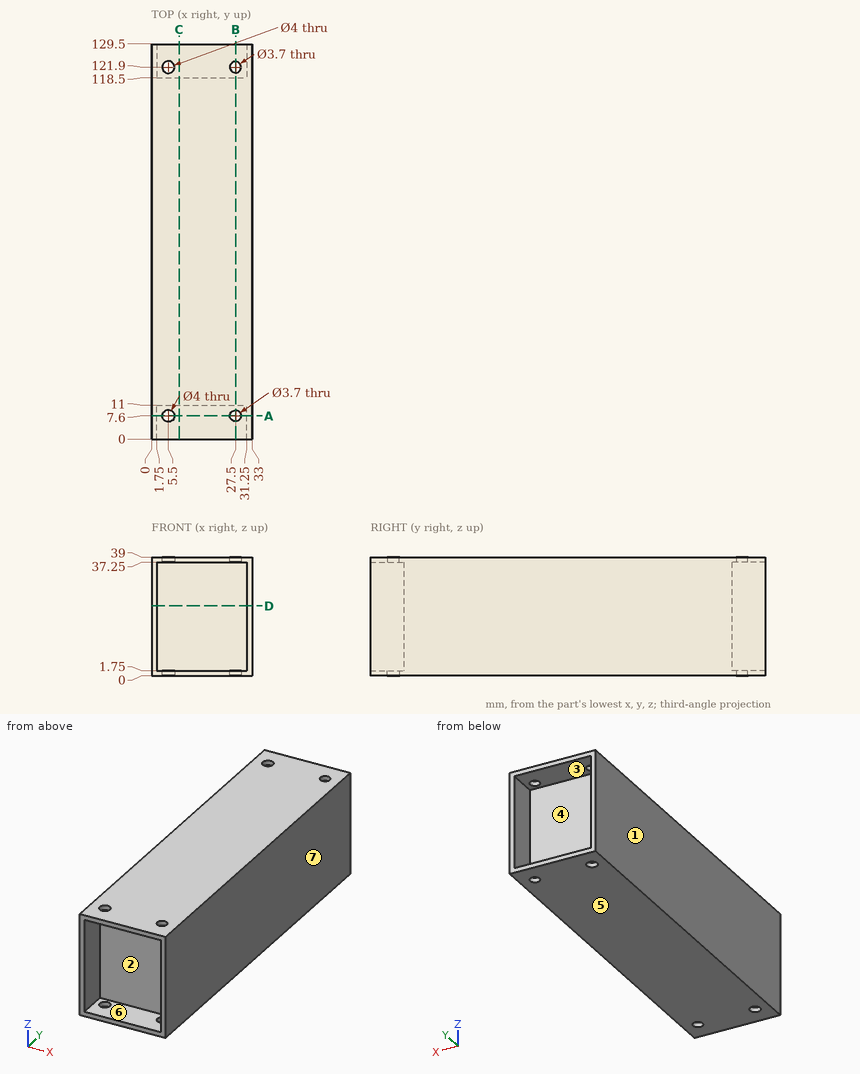
Can you work these out from the drawing? Everything is in mm from the part's minimum corner. A direction names the side the tool comes from. Coordinates: 2 decimals unless noted, no trailing zeros. Order: outer loops, then holes, each group sorted by start corner. A loop starts at its lowest first (then second) coordinate and runs counter-clockwise, first axis right, second up. Notation, with made-up numbers: (68.25, -36.5) -> (117.25, -36.5) arc R20 ccw to (117.25, -32.5) -> close; hole circle Ø11 at (70.5, 56.25). An arc over 180 degrees is marked (long way). Use one line per item in the form item = value.
Q1. Imagine slicing it at B-B, the plane x = 27.5. List the corners of the cut face in (y, z) for me.
From the geometry:
outline = (0, 0) -> (5.75, 0) -> (5.75, 1.75) -> (0, 1.75) -> close; (0, 37.25) -> (5.75, 37.25) -> (5.75, 39) -> (0, 39) -> close; (9.45, 0) -> (120.05, 0) -> (120.05, 1.75) -> (118.5, 1.75) -> (118.5, 37.25) -> (120.05, 37.25) -> (120.05, 39) -> (9.45, 39) -> (9.45, 37.25) -> (11, 37.25) -> (11, 1.75) -> (9.45, 1.75) -> close; (123.75, 0) -> (129.5, 0) -> (129.5, 1.75) -> (123.75, 1.75) -> close; (123.75, 37.25) -> (129.5, 37.25) -> (129.5, 39) -> (123.75, 39) -> close
Q2. Imagine slicing it at D-D, the plane z = 23. List the corners of the cut face in (x, y) for me, then the cut area to 3 significant figures.
From the geometry:
outline = (0, 0) -> (1.75, 0) -> (1.75, 11) -> (31.25, 11) -> (31.25, 0) -> (33, 0) -> (33, 129.5) -> (31.25, 129.5) -> (31.25, 118.5) -> (1.75, 118.5) -> (1.75, 129.5) -> (0, 129.5) -> close
area = 3,620 mm²
Q3. We'd pull the mould along Z, two halves only. Please class the marked faces 4, 5, 6 and 7: released by +Z, released by -Z, zero draft, split by the parting line, or undercut.
From the geometry:
face_4 = undercut
face_5 = released by -Z
face_6 = undercut
face_7 = zero draft
Q4. Which directions (+Z, -Z, +X, -X, +Y, -Y) give clear straight access to the entire face, cutting with the end or side of a thin tool? Please do the marked faces 1, 2 and 3.
From the geometry:
face_1 = +Z, -Z, -X, +Y, -Y
face_2 = -Y
face_3 = +Y
Q5. Imagine slicing it at C-C, the plane x = 9. List the corners of the cut face in (y, z) for me, then the cut area to 3 significant figures.
From the geometry:
outline = (0, 0) -> (129.5, 0) -> (129.5, 1.75) -> (118.5, 1.75) -> (118.5, 37.25) -> (129.5, 37.25) -> (129.5, 39) -> (0, 39) -> (0, 37.25) -> (11, 37.25) -> (11, 1.75) -> (0, 1.75) -> close
area = 4,270 mm²
Q6. Will this pin go through, and if not, where does the flat tip stop? P1, Ø9, axis at x = 16.5, z = 15.5, coming from the +Y side.
From the geometry:
P1 = 118.5
Q7. I need wall thicknesses on L1, parallel to Y at x = 27.5, z = 38.4; L2, parallel to Y at x = 5.5, z = 37.7; L3, parallel to X at y = 7.6, z = 37.85. Which ranges of each line are inside material? Lowest first, please.
From the geometry:
L1 = 0 to 5.75, 9.45 to 120.05, 123.75 to 129.5
L2 = 0 to 5.6, 9.6 to 119.9, 123.9 to 129.5
L3 = 0 to 3.5, 7.5 to 25.65, 29.35 to 33
Q8. Imagine slicing it at A-A, the plane y = 7.6. List the corners of the cut face in (x, z) for me.
From the geometry:
outline = (0, 0) -> (3.5, 0) -> (3.5, 1.75) -> (1.75, 1.75) -> (1.75, 37.25) -> (3.5, 37.25) -> (3.5, 39) -> (0, 39) -> close; (7.5, 0) -> (25.65, 0) -> (25.65, 1.75) -> (7.5, 1.75) -> close; (7.5, 37.25) -> (25.65, 37.25) -> (25.65, 39) -> (7.5, 39) -> close; (29.35, 0) -> (33, 0) -> (33, 39) -> (29.35, 39) -> (29.35, 37.25) -> (31.25, 37.25) -> (31.25, 1.75) -> (29.35, 1.75) -> close
